Input: part model. Units: mm. Frame: model coordinates. A direction names the side the tool comes from. Coordinates: 2 decimals unless noted, no trailing zeros. Loops run counter-clockwise (first coordinate to the right, second up) from the corner with the lowest first, then second, coordinate; pieces in that order, holes last. Notation, with made-up numbers: (22, 42) - (69, 42) arc R12 ccw to (69, 48) - close; hole circle Ø2 at (-18.75, 84.25). An arc over 180 degrees is marked (long way). Use a Markdown table: item, result. Add a question column.
1. Section query A-A on z = 49.5. Return the cut outline in (x, y), then the cut area to 3 significant figures.
2. Section query C-C on x = 321. Return the cut outline in (y, z), then the cut area to 3 significant figures.
3. Access query for faces 1 (the face through (-7.6, 2.8, 5.7)), 2 (the face through (227.03, 3.639, 308.776)), 3 (the face through (7, -6.42, 111.54)). Directions: +Z, -Z, +X, -X, +Y, -Y. A direction counts if a zero-diameter tool reaches every point of the face in a straight line with its end or side. Return the directions, or none.
4. Section query D-D on z = 245. State how many separate pieces and enclosed holes the cut face has, then the cut area to 3 significant figures.
5. Contact query for flat-ended pins moving along their axis: P1, Ø2, axis at y = 1.5, z = 275, coming from the -X side; P2, Ø3, axis at x = 119.5, y = 7, coming from the +Z side; P3, Ø9.5, axis at x = 0, y = 0, coming from the +Z side; P4, Ø1, axis at x = 127, y = 0.5, coming from the +Z side. Output: stop coordinate, or through.
6. Draft query along Z for faces 4 (the face through (227.03, -2.373, 307.535)), 5 (the face through (442.4, 2.8, 5.7)), 6 (the face through (458.776, 3.639, 108.46)). Return one class per face: released by +Z, released by -Z, zero draft, split by the parting line, or undercut.
7. Ray query, L1, parallel to X at y = 0, z = 166; L2, parallel to X at y = 1, z = 96.5; L3, parallel to Y at x = 450, z = 138.5. Return the intervals inside material, ascending. Write a range as [from, to].
Solid Edge part; units mm, degrees
sketch "Sketch1" plane through (0, 0, 0) normal (0, -1, 0) x (1, 0, 0)
  line L0 (0, 0) -> (0, 220)
  arc A0 (0, 220) -> (80, 300) centre (80, 220) cw
  line L1 (80, 300) -> (370, 300)
  arc A1 (370, 300) -> (450, 220) centre (370, 220) cw
  line L2 (450, 220) -> (450, 0)
sketch "Sketch2" plane through (0, 0, 0) normal (0, 0, -1) x (-1, 0, 0)
  circle A0 centre (0, 0) radius 9.5
sweep "SweptProtrusion_1" add profiles "Sketch2" path "Sketch1"
shell "Thinwall_1" thickness 1.6 removed faces 4 at (6.5233, -6.1433, 0) at (443.4767, -6.1433, 0) at (6.5233, -6.1433, 0) at (443.4767, -6.1433, 0)
hole "Hole_1" at (0, 0, 0) direction (0, -1, 0) diameter 19 end through all both ways yes
hole "Hole1" at (450, 0, 0) direction (0, -1, 0) diameter 19 end through all both ways yes
properties material "Aluminum, 1060"
Resolved:
| question | item | result |
|---|---|---|
| 1 | outline | circle Ø19 at (0, 0); circle Ø19 at (450, 0); hole circle Ø15.8 at (0, 0); hole circle Ø15.8 at (450, 0) |
| 1 | area | 175 mm² |
| 2 | outline | circle Ø19 at (0, 300); hole circle Ø15.8 at (0, 300) |
| 2 | area | 87.5 mm² |
| 3 | face 1 | -Z, +Y, -Y |
| 3 | face 2 | none |
| 3 | face 3 | -Z |
| 4 | separate pieces | 2 |
| 4 | enclosed holes | 2 |
| 4 | area | 184 mm² |
| 5 | P1 | x = 8.75 |
| 5 | P2 | z = 307.75 |
| 5 | P3 | z = 268.45 |
| 5 | P4 | z = 309.5 |
| 6 | face 4 | undercut |
| 6 | face 5 | released by -Z |
| 6 | face 6 | zero draft |
| 7 | L1 | [-9.5, -7.9], [7.9, 9.5], [440.5, 442.1], [457.9, 459.5] |
| 7 | L2 | [-9.45, -7.84], [7.84, 9.45], [440.55, 442.16], [457.84, 459.45] |
| 7 | L3 | [-9.5, -7.9], [7.9, 9.5] |
